Source: CAD feature listing. Evaluate the final solid. Frame: model axes, mm. A direction names the side the tool comes from. Round coordinates to 2 decimals unless told otherwise and drop trailing zeros. Order: outer loops, then holes, each group sorted by start corner. A loop starts at its lowest first (then second) coordinate and runs counter-clockwise, first axis right, second up. Notation, with made-up numbers: (-22.5, -33.5) -> (-9.5, -33.5) arc R32 ccw to (-9.5, -0.5) -> close; hole circle Ø7 at (8, 78). An arc over 180 degrees is marked (long way). Answer as CSV lines item,"result". Start each with the question number.
(1) Section query D-D (x = 12). Output: boundary loops of the cut face in (y, z), plus the area to 3 significant figures.
(2) Section query C-C (y = 25.5). Output: boundary loops of the cut face in (x, z), plus the area to 3 significant figures.
(3) Pull-direction query (Z, two-part tool) for faces 1 (the flat face through (6, 0, 0)), 2 (the flat face through (-0.086, 78.607, 5.643)), 3 (the cylindrical face through (-14.985, 37.961, -0.66)); classes: +Z half, -Z half, draft (parallel to the pull), parting line (faces both ways), or undercut.
(4) Section query A-A (x = 0). Output: boundary loops of the cut face in (y, z).
(5) Set-up query: faces 4 (the flat face through (-0.086, 78.607, -5.643)), 5 (the flat face through (14, 77, -6)), 6 (the flat face through (-5.15, 38, 0)). Return all of +Z, -Z, +X, -X, +Y, -Y with unobstructed straight access to the full face (end or side cutting, diameter ignored); none if empty.
(6) Contact query for flat-ended pins moving along their axis: P1, Ø5, axis at x = 14, z = -8, coming from the -Y side; P2, Ø8, axis at y = 57, z = -1, coming from the +X side; P3, Ø8, axis at x = -1, y = 33.5, coming from the +Z side; P4, Ø6, axis at y = 62.5, z = -5.5, coming from the -X side. Output: stop coordinate, or through.
(7) Line query: line 1 along Z through (x, y) = (0.5, 12); line 2 along X through (y, z) = (69.5, -3.5); line 3 along Z through (x, y) = (-2, 46). Output: solid intervals per line, ascending. Write a range as from..to.
(8) Section query B-B (z = 0). Output: boundary loops of the cut face in (x, y).
```python
from build123d import *

# Parameters (mm, degrees)
SKETCH_1_R          = 15
SKETCH_1_W          = 10.3
SKETCH_1_H          = 10.3
EXTRUDE_1_DEPTH     = 80
SKETCH1_R           = 19
SKETCH1_W           = 10.3
SKETCH1_H           = 10.3
BOSS_EXTRUDE1_DEPTH = 3
CHAMFER1_SIZE       = 1
CHAMFER1_SIZE2      = 2.747477419


with BuildPart() as part:
    # Эскиз1 → Бобышка-Вытянуть1 (new body)
    with BuildSketch(Plane(origin=(0, 0, 0), x_dir=(1, 0, 0), z_dir=(0, 1, 0))):
        Circle(SKETCH_1_R)
        Rectangle(SKETCH_1_W, SKETCH_1_H, mode=Mode.SUBTRACT)
    extrude(amount=EXTRUDE_1_DEPTH)

    # Sketch1 → Boss-Extrude1 (add)
    with BuildSketch(Plane(origin=(0, 80, 0), x_dir=(1, 0, 0), z_dir=(0, 1, 0))):
        Circle(SKETCH1_R)
        Rectangle(SKETCH1_W, SKETCH1_H, mode=Mode.SUBTRACT)
    extrude(amount=-BOSS_EXTRUDE1_DEPTH)

    # Chamfer1
    chamfer1_edges = [part.edges().sort_by_distance(p)[0] for p in [
        (0, 80, -5.15),
        (-5.15, 80, 0),
        (0, 80, 5.15),
        (5.15, 80, 0),
    ]]
    chamfer1_side = [part.faces().sort_by_distance(p)[0] for p in [
        (-18.462598846, 80, 0),
    ]]
    chamfer(chamfer1_edges, length=CHAMFER1_SIZE, length2=CHAMFER1_SIZE2, reference=chamfer1_side[0])


solid = part.part
```
Answer block:
1,outline,"(0, -9) -> (77, -9) -> (77, -14.73) -> (80, -14.73) -> (80, 14.73) -> (77, 14.73) -> (77, 9) -> (0, 9) -> close"
1,area,"1,470 mm2"
2,outline,"circle Ø30 at (0, 0); hole (-5.15, -5.15) -> (5.15, -5.15) -> (5.15, 5.15) -> (-5.15, 5.15) -> close"
2,area,"601 mm2"
3,face 1,"draft"
3,face 2,"undercut"
3,face 3,"parting line"
4,outline,"(0, -15) -> (77, -15) -> (77, -19) -> (80, -19) -> (80, -6.15) -> (77.25, -5.15) -> (0, -5.15) -> close; (0, 5.15) -> (77.25, 5.15) -> (80, 6.15) -> (80, 19) -> (77, 19) -> (77, 15) -> (0, 15) -> close"
5,face 4,"+Y"
5,face 5,"-Y"
5,face 6,"+Y, -Y"
6,P1,"y = 0"
6,P2,"x = 15"
6,P3,"z = 15"
6,P4,"x = -14.79"
7,line 1,"-14.99..-5.15, 5.15..14.99"
7,line 2,"-14.59..-5.15, 5.15..14.59"
7,line 3,"-14.87..-5.15, 5.15..14.87"
8,outline,"(-19, 77) -> (-15, 77) -> (-15, 0) -> (-5.15, 0) -> (-5.15, 77.25) -> (-6.15, 80) -> (-19, 80) -> close; (5.15, 0) -> (15, 0) -> (15, 77) -> (19, 77) -> (19, 80) -> (6.15, 80) -> (5.15, 77.25) -> close"
